from build123d import *

# Parameters (mm, degrees)
EXTRUDE1_DEPTH          = 11.1125
EXTRUDE1_DEPTH_BACK     = 11.1125
SKETCH12_R              = 6.6675
CUT_EXTRUDE4_DEPTH      = 41.26308225
CUT_EXTRUDE4_DEPTH_BACK = 41.26308225
SKETCH10_R              = 4.7625
CHAMFER1_SIZE           = 0.47625


with BuildPart() as part:
    # Sketch7 → Revolve3 (revolve)
    with BuildSketch(Plane.XY):
        with BuildLine():
            Line((0, 37.2999), (0, 16.6751))
            ThreePointArc((0, 16.6751), (10.3124, 26.9875), (0, 37.2999))
        make_face()
    revolve(axis=Axis((0, 0, 0), (0, 1, 0)))

    # Sketch12 → Extrude1 (add, two sides: drawn at the far end of the back side and taken through both)
    with BuildSketch(Plane.XY.offset(-EXTRUDE1_DEPTH_BACK)):
        with Locations((0, 26.9875)):
            Circle(SKETCH12_R)
    extrude(amount=EXTRUDE1_DEPTH + EXTRUDE1_DEPTH_BACK)

    # Sketch10 → Cut-Extrude4 (cut, two sides: drawn at the far end of the back side and taken through both)
    with BuildSketch(Plane.XY.offset(-CUT_EXTRUDE4_DEPTH_BACK)):
        with Locations((0, 26.9875)):
            Circle(SKETCH10_R)
    extrude(amount=CUT_EXTRUDE4_DEPTH + CUT_EXTRUDE4_DEPTH_BACK, mode=Mode.SUBTRACT)

    # Chamfer1
    chamfer1_edges = [part.edges().sort_by_distance(p)[0] for p in [
        (-4.7625, 26.9875, -11.1125),
        (-4.7625, 26.9875, 11.1125),
    ]]
    chamfer(chamfer1_edges, length=CHAMFER1_SIZE)


solid = part.part
CAD build for the part. Positions are in the model's coordinates, mm. A direction names the side the tool comes from. Coordinates: 2 decimals unless noted, no trailing zeros. Write each loop counter-clockwise with the first axis right and the second up, starting at its lowest first coordinate (ties: lowest second). Pieces come first, ordered by that corner, then holes. Notation, with made-up numbers: (-17, 70) - (-11, 70) arc R18 ccw to (-11, 103) - close; hole circle Ø5 at (24.5, -30.75). An arc over 180 degrees is marked (long way). Use a Markdown table: item, result. Add a question column.
Item 1: Flat gauge pins, fed straight in: pin 1 (3 mm diameter, centred on x = 4, z = 6.5, fed in from -Y); pin 2 (8 mm diameter, centred on x = 7.5, z = -5, fed in from +Y); pin 3 (1 mm diameter, centred on x = -2, z = 3, fed in from -Y). Where does each tip first touch, or does it go through?
Item 2: Band-saw the part on D-D, the plane x = -8.5. Give the cut face in (y, z), and give its area (3 significant figures).
Item 3: Drill centre lines: L1, parallel to X at y = 30.5, z = 6.25; L2, parallel to Y at x = 0, z = 3 (3 decimals); L3, parallel to Y at x = -2.75, z = 4.25. Where is each one in solid material? Low to high. Write a range as from..to.
Item 4: Band-saw the part on C-C, the plane y = 18.75. Give the cut face in (x, z), and give its area (3 significant figures).
Item 5: Mould opens along Y. For faces 3 (the face through (-0.87, 33.6, -9.51)), 4 (the face through (-0.62, 31.71, -0.15)), 5 (the face through (-0.03, 21.59, 11.112)) say: pulls with the +Y half, pulls with the -Y half, needs draft (parallel to the pull), parting line crosses it, or undercut.
Item 6: Band-saw the part on B-B, the plane z = 3.75. Give the cut face in (x, y) (1 decimal), and give its area (3 significant figures).
Item 7: 3-axis set-ups, long thin cutter, end or side, ignore diameter. For faces 1 (the face through (-0.03, 21.59, -11.112)), 2 (the face through (-0.87, 33.6, 9.47)): which of +Z, -Z, +X, -X, +Y, -Y reach the whole face in a straight line?
Numbers:
| question | item | result |
|---|---|---|
| 1 | pin 1 | y = 18.7 |
| 1 | pin 2 | y = 36 |
| 1 | pin 3 | y = 17.15 |
| 2 | outline | circle Ø11.68 at (26.99, 0) |
| 2 | area | 107 mm2 |
| 3 | L1 | -7.41..-3.22, 3.22..7.41 |
| 3 | L2 | 17.121..22.225, 31.75..36.854 |
| 3 | L3 | 18..23.1, 30.88..35.97 |
| 4 | outline | circle Ø12.41 at (0, 0) |
| 4 | area | 121 mm2 |
| 5 | face 3 | parting line crosses it |
| 5 | face 4 | undercut |
| 5 | face 5 | needs draft |
| 6 | outline | circle Ø19.2 at (0, 27); hole circle Ø9.5 at (0, 27) |
| 6 | area | 219 mm2 |
| 7 | face 1 | -Z, +X, -X, +Y, -Y |
| 7 | face 2 | +Z |
